Autodesk Fusion 360 part; units mm, degrees
sketch "Skizze13" plane through (0, 0, 0) normal (0, 0, 1) x (1, 0, 0)
  circle A0 centre (0, 0) radius 80
extrude "Extrusion17" add sketch "Skizze13" along normal blind 10 makes body 1
fillet "Abrundung5" radius 2 1 edges at (-74.5862, -28.9292, 10) on bodies 1
sketch "Skizze14" plane through (0, 0, 0) normal (0, 1, 0) x (1, 0, 0)
  line L0 (25, 0) -> (-17.2618, -90.6308) construction
ref_plane "Arbeitsebene5" through (-17.2618, 0, 90.6308) normal (-0.4226, 0, 0.9063) x (0, -1, 0)
sketch "Skizze15" plane through (-17.2618, 0, 90.6308) normal (-0.4226, 0, 0.9063) x (0, -1, 0)
  circle A0 centre (0, 0) radius 24
  circle A1 centre (0, 0) radius 21.5
extrude "Extrusion20" add sketch "Skizze15" against normal blind 110 separate body contours A0 | A1 makes body 2
combine "Kombinieren3" operation add target body 1 tool bodies 2
extrude "Extrusion21" cut sketch "Skizze15" against normal blind 17 bodies 1
fillet "Abrundung6" radius 4 1 edges at (46.818, 0, 10) on bodies 1
sketch "Skizze16" plane through (-17.2618, 0, 90.6308) normal (-0.4226, 0, 0.9063) x (0, -1, 0)
  circle A0 centre (0, 0) radius 17
extrude "Extrusion22" cut sketch "Skizze16" against normal blind 160 bodies 1
sketch "Skizze17" plane through (0, 0, 0) normal (0, 0, 1) x (1, 0, 0)
  circle A0 centre (0, 0) radius 160
extrude "Extrusion23" cut sketch "Skizze17" against normal blind 110 bodies 1
ref_plane "Arbeitsebene6" through (90, 0, 0) normal (1, 0, 0) x (0, 1, 0)
sketch "Skizze18" plane through (90, 0, 0) normal (1, 0, 0) x (0, 0, -1)
  circle A0 centre (-5, 0) radius 3.5
extrude "Extrusion24" cut sketch "Skizze18" against normal blind 70 bodies 1
chamfer "Fase3" distance 0.7 angle 45 3 edges at (41.122, -3.4937, 4.7932) (79.9365, 0.0176, 8.5) (80, 0, 1.5) on bodies 1
equation "base_plate_diameter = 160 mm"
equation "base_plate_height = 10 mm"
equation "base_plate_rounding = 2 mm"
equation "arm_outer_diameter = 48 mm"
equation "ring_inner_diameter = 43 mm"
equation "ring_extrude_depth = 17 mm"
equation "foot_leg_bore_diameter = 34 mm"
equation "leg_length = 100 mm"
equation "leg_angle = 115 deg"
equation "leg_offset = 25 mm"
equation "leg_plate_rounding = 4 mm"
equation "cable_hole_offset = 90 mm"
equation "cable_hole_depth = 70 mm"
equation "cable_hole_diameter = 7 mm"
equation "cable_hole_height = 5.0 mm"
equation "cable_hole_chamfer = 0.7 mm"
equation "d81 = base_plate_height"
equation "d84 = base_plate_rounding"
equation "d95 = leg_plate_rounding"
equation "d96 = -leg_length - base_plate_height - 50 mm"
equation "d104 = cable_hole_chamfer"
The model under review builds one solid part; all positions refer to its coordinate system, in mm. A direction names the side the tool comes from. Give positions to 0.01 mm unless a question says otherwise; leave off trailing zeros.
(1) Tool access review of faces 4 (the flat face through (-6.753, 21.445, 76.774)), 5 (the cylindrical face through (-17.34, 78.1, 3.94)): name each direction out of +Z, -Z, +X, -X, +Y, -Y from which nothing blocks a thin tool from reaching the whole face with its end or side.
(2) The part is to be moulded in two halves that separate along Y. For faces 1 (the cylindrical face through (60.168, 0.154, 8.497)), 2 (the flat face through (-1, 1, 0)), 3 (the cylindrical face through (-21.18, -19.86, 79.55)), say which applies: released by +Y, released by -Y, zero draft, split by the parting line, or undercut.
(3) To check wall thickness, follow L1, parallel to Z at x = 69.5, y = 0; L2, parallel to Z at x = -39.5, y = 7; L3, parallel to Z at x = -36, y = 3.5. State the ranges of each line that lie inside material, in increasing order.
(4) For P1, Ø8, axis at x = 56.5, y = -14, coming from the +Z side; P2, Ø2, axis at y = -45, z = 10.5, coming from the +X side; P3, Ø6, axis at y = -20, z = 70, coming from the +X side, all flat-tipped, find the tip position at first contact; note any pin that passes through.
Returned:
1. face 4: none
1. face 5: +Z, -Z
2. face 1: undercut
2. face 2: zero draft
2. face 3: split by the parting line
3. L1: z = 0 to 1.5, 8.5 to 10
3. L2: z = 0 to 10
3. L3: z = 0 to 10, 80.62 to 81.89
4. P1: stops at z = 10
4. P2: stops at x = 65.47
4. P3: stops at x = 11.33
